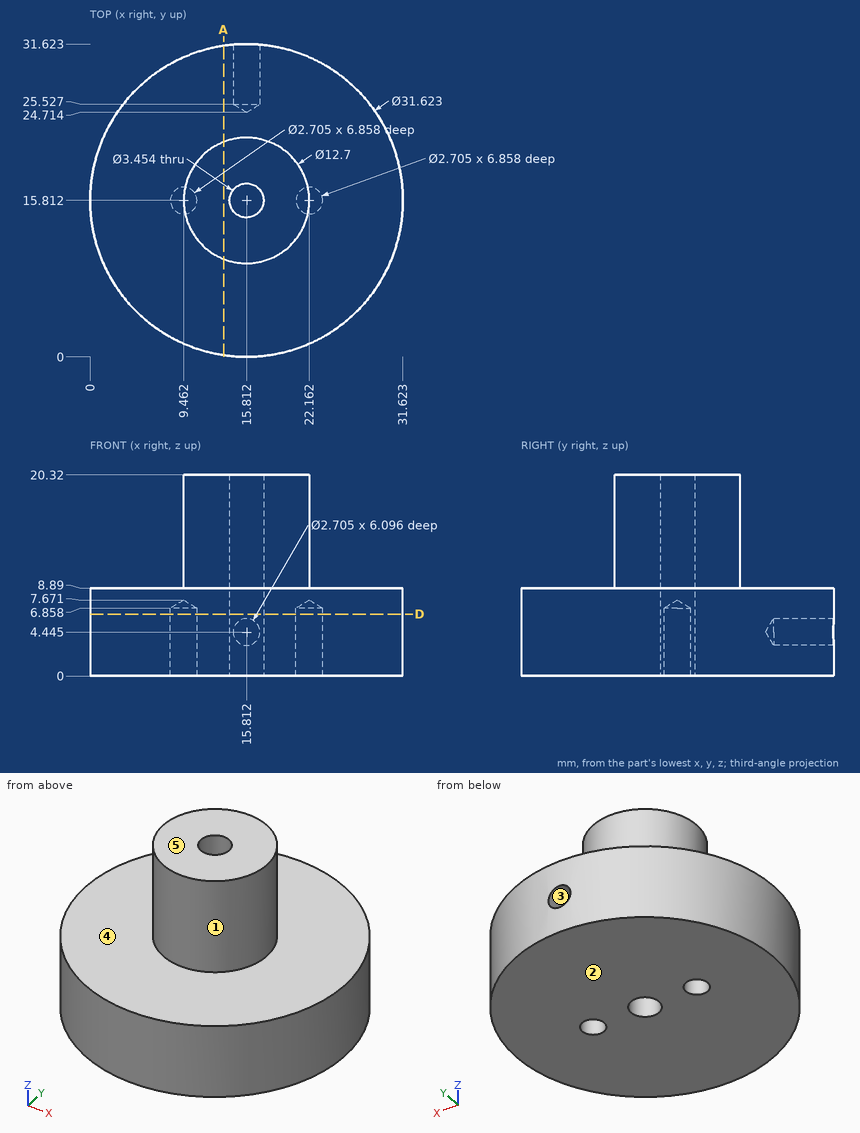
Answer from the drawing. Dimensions are ordinates in mm from the lowest x, y and z of the part. A direction names the side the tool comes from. Coordinates: 2 decimals unless noted, no trailing zeros. Write each loop counter-clockwise with the first axis right and the second up, starting at its lowest first coordinate (ties: lowest second). Pieces come first, ordered by that corner, then holes. Notation, with made-up numbers: M -23,-1.75 L 3,-1.75 A16 ccw 3,14.25 Z; hole C 50.5,5.25 d3. An arc over 180 degrees is marked long. Use a Markdown table: item, result.
Q1. The part is cut by section D-D, the plane z = 6.25. Write down the section's boundary in (x, y) (1 decimal).
Answer block:
| item | result |
|---|---|
| outline | C 15.8,15.8 d31.6; hole C 9.5,15.8 d2.7; hole C 15.8,15.8 d3.5; hole C 22.2,15.8 d2.7 |
Q2. The part is cut by section A-A, the plane x = 13.5. Write down the section's boundary in (y, z) (1 decimal).
Answer block:
| item | result |
|---|---|
| outline | M 0.2,0 L 31.5,0 L 31.5,8.9 L 21.7,8.9 L 21.7,20.3 L 9.9,20.3 L 9.9,8.9 L 0.2,8.9 Z |
Q3. Determine the mould class of the marked faces 1, 2 and 3 for opening direction X: released by +X, released by -X, zero draft, split by the parting line, or undercut.
Answer block:
| item | result |
|---|---|
| face 1 | split by the parting line |
| face 2 | zero draft |
| face 3 | undercut |
Q4. Each of these flat-tipped pins is pushed along its axis until it touches: pin 1 Ø3 at (x, z) = (22, 13) entering from +Y (1 decimal); pin 2 Ø1.5 at (x, z) = (16, 13.5) entering from -Y; pin 3 Ø2 at (y, z) = (20, 14.5) entering from -X. Where does it stop, or does it pass through?
Answer block:
| item | result |
|---|---|
| pin 1 | stops at y = 20.1 |
| pin 2 | stops at y = 9.46 |
| pin 3 | stops at x = 10.32 |
Q5. Which of the six approach directions +Z, -Z, +X, -X, +Y, -Y give full straight-line access (tool end or side, diameter ignored) to the marked faces 4 and 5?
Answer block:
| item | result |
|---|---|
| face 4 | +Z |
| face 5 | +Z, +X, -X, +Y, -Y |
Q6. Straight lines are drawn through the part: L1, parallel to Y at x = 16, z = 14.25 (1 decimal); L2, parallel to Z at x = 14.5, y = 4; L3, parallel to X at y = 16.5, z = 6.25 (1 decimal). For each, find the intervals that lie inside material, in ascending order. Write a range as [from, to].
Answer block:
| item | result |
|---|---|
| L1 | y = [9.5, 14.1], [17.5, 22.2] |
| L2 | z = [0, 8.89] |
| L3 | x = [0, 8.3], [10.6, 14.2], [17.4, 21], [23.3, 31.6] |
